Geometry check sheet. Reference: the model listing, model coordinates, mm. Face numbers are marked on the shaded views. Give positions to 0.01 mm unless a question says otherwise; leave off trailing zeros. Loops run counter-clockwise (first coordinate to the right, second up) from the corner with the lowest first, then second, coordinate; pieces in that order, holes last. Notation, with made-up numbers: (-16.75, -25.75) -> (-2.75, -25.75) arc R24 ccw to (-2.75, 13.25) -> close; hole circle Ø5 at (71, -36.5). An arc over 180 degrees is marked (long way). One line per question, with ' | ' between items.
from build123d import *

# Parameters (mm, degrees)
BOSS_EXTRUDE1_DEPTH = 50
SKETCH5_R           = 65
CUT_EXTRUDE3_DEPTH  = 50
SKETCH4_R           = 160
CUT_EXTRUDE4_DEPTH  = 50


with BuildPart() as part:
    # Sketch1 → Boss-Extrude1 (new body)
    with BuildSketch(Plane(origin=(0, 0, 0), x_dir=(1, 0, 0), z_dir=(0, 1, 0))):
        with BuildLine():
            ThreePointArc((-79.615153419, -29.772929752), (-76.142301846, -140.554949646), (-98.232528839, -249.167741256))
            ThreePointArc((-98.232528839, -249.167741256), (-2.78801704, -579.97840693), (102.857311412, -252.28279217))
            ThreePointArc((102.857311412, -252.28279217), (79.272553954, -140.112834924), (81.083403738, -25.504541524))
            ThreePointArc((81.083403738, -25.504541524), (-2.256928059, 84.970031633), (-79.615153419, -29.772929752))
        make_face()
    extrude(amount=BOSS_EXTRUDE1_DEPTH)

    # Sketch5 → Cut-Extrude3 (cut)
    with BuildSketch(Plane(origin=(0, 50, 0), x_dir=(1, 0, 0), z_dir=(0, 1, 0))):
        with Locations(Location((0, 0, 0), (0, 0, 270))):
            Circle(SKETCH5_R)
    extrude(amount=-CUT_EXTRUDE3_DEPTH, mode=Mode.SUBTRACT)

    # Sketch4 → Cut-Extrude4 (cut)
    with BuildSketch(Plane(origin=(0, 50, 0), x_dir=(1, 0, 0), z_dir=(0, 1, 0))):
        with Locations(Location((0, -400, 0), (0, 0, 270))):
            Circle(SKETCH4_R)
    extrude(amount=-CUT_EXTRUDE4_DEPTH, mode=Mode.SUBTRACT)


solid = part.part
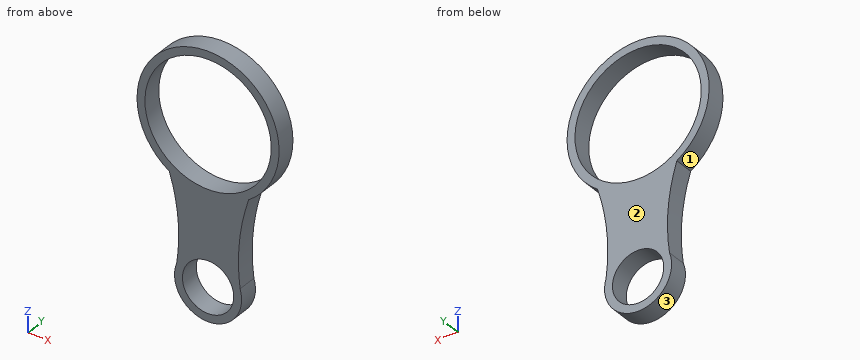
Item 1: Sectioned sample at B-B (z = 0). Record the cut outline in (x, y), plus the area to 3 significant figures.
Result:
outline: (-85, 0) -> (-65, 0) -> (-65, 50) -> (-85, 50) -> close; (65, 0) -> (85, 0) -> (85, 50) -> (65, 50) -> close | area: 2,000 mm2
Item 2: Release check for a two-part mould opening along Z. For the marked faces 1, 2 and 3 record: pulls with the +Z half, pulls with the -Z half, needs draft (parallel to the pull), parting line crosses it, or undercut.
Result:
face 1: parting line crosses it | face 2: needs draft | face 3: undercut
Item 3: Sectioned sample at C-C (y = 8.5). Record the cut outline in (x, z).
Result:
outline: (-98.23, 249.17) arc R478.84 cw to (-79.62, 29.77) arc R85 ccw (long way) to (81.08, 25.5) arc R514.98 cw to (102.86, 252.28) arc R180 ccw (long way) to start; hole circle Ø320 at (0, 400); hole circle Ø130 at (0, 0)
Item 4: Sectioned sample at A-A (x = 0). Record the cut outline in (y, z).
Result:
outline: (0, -85) -> (50, -85) -> (50, -65) -> (0, -65) -> close; (0, 65) -> (50, 65) -> (50, 240) -> (0, 240) -> close; (0, 560) -> (50, 560) -> (50, 580) -> (0, 580) -> close
Item 5: Depth check by flat-ended pin: pin 1 Ø1.5 at (y, z) = (28, 478) entering from -X; pin 2 Ø1.5 at (y, z) = (42.5, 469) entering from -X; pin 3 Ø10 at (y, z) = (39.5, 21) entering from -X. Enter the tip coordinate at first touch or a pass-through.
Result:
pin 1: x = -162.58 | pin 2: x = -166.56 | pin 3: x = -83.48
Item 6: Sectioned sample at D-D (z = 294.5). Record the cut outline in (x, y).
Result:
outline: (-145.84, 0) -> (-120.29, 0) -> (-120.29, 50) -> (-145.84, 50) -> close; (120.29, 0) -> (145.84, 0) -> (145.84, 50) -> (120.29, 50) -> close
Item 7: Scan lines: probe 1 along X at (y, z) = (37, 400); probe 2 along X at (y, z) = (30, 0); probe 3 along Z at (x, y) = (-5.5, 16.5). Record each from-to range of solid material in increasing order.
Result:
probe 1: -180 to -160, 160 to 180 | probe 2: -85 to -65, 65 to 85 | probe 3: -84.82 to -64.77, 64.77 to 240.09, 559.91 to 579.92
